Here's the drawing with two shaded views (mm, measured from the low corner). I have some questions. Give positions to 0.01 mm unless a question says otherwise; leave off trailing zeros. Write each loop counter-clockwise with the first axis right and the second up, starting at its lowest first coordinate (ties: lowest second). Pieces come first, ordered by that corner, then holes. Notation, with made-up numbers: M 72.25,22 L 102.25,22 A3 ccw 102.25,27 Z; hole C 76,88 d7. An arc over 180 degrees is marked long. Use one line per item in the form item = value.
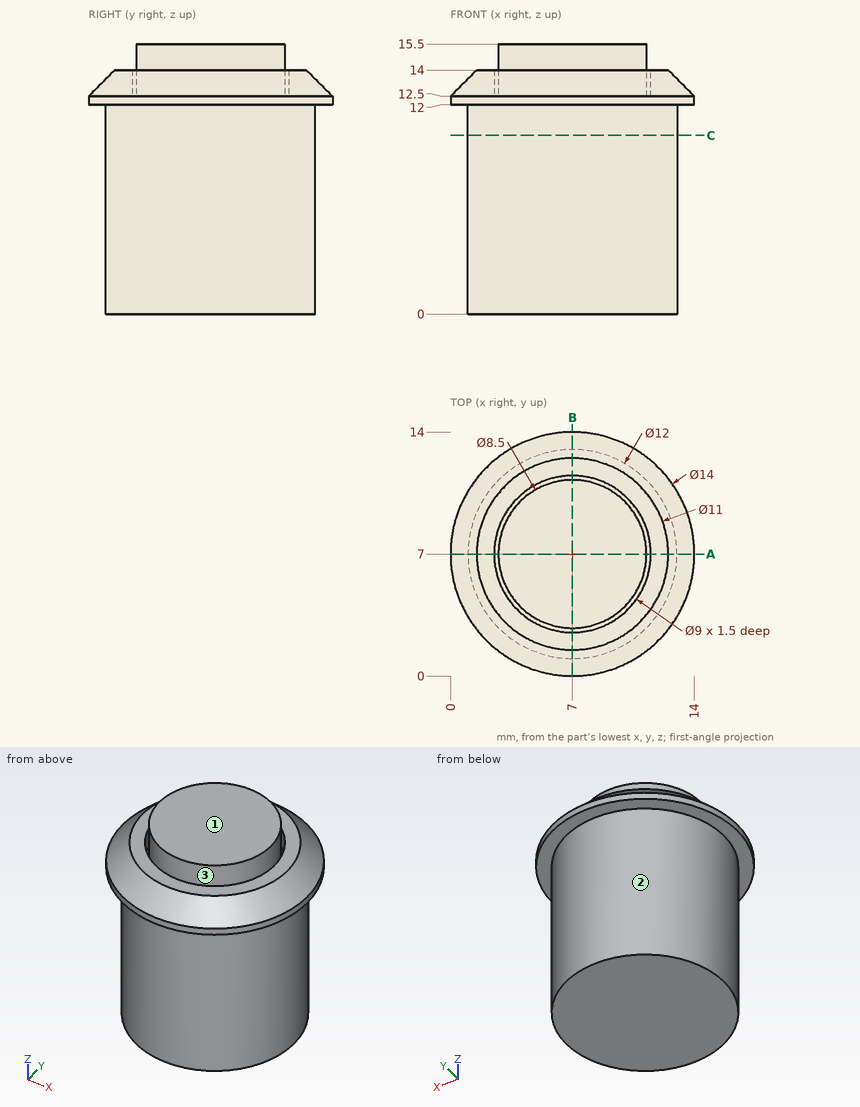
1) If I drill on L1, parallel to Y at x = 7, z = 13.15; L2, parallel to Y at x = 7, z = 12.95; L3, parallel to Z at x = 3, y = 4, over which ranges is the centre line in solid material (lowest first)?
Checked values:
L1 = 0.65 to 2.5, 2.75 to 11.25, 11.5 to 13.35
L2 = 0.45 to 2.5, 2.75 to 11.25, 11.5 to 13.55
L3 = 0 to 14
2) I want a section at A-A, the plane y = 7. Please give me the cut outline in (x, z).
Checked values:
outline = M 0,12 L 1,12 L 1,0 L 13,0 L 13,12 L 14,12 L 14,12.5 L 12.5,14 L 11.5,14 L 11.5,12.5 L 11.25,12.5 L 11.25,15.5 L 2.75,15.5 L 2.75,12.5 L 2.5,12.5 L 2.5,14 L 1.5,14 L 0,12.5 Z
3) I want a section at C-C, the plane z = 10.25. Please give me the cut outline in (x, y), plus the area to 3 significant figures.
Checked values:
outline = C 7,7 d12
area = 113 mm2
4) Thinking about a two-plate mould opening in X: for the marked faces 1, 2 and 3, which applies, released by +X, released by -X, zero draft, split by the parting line, or undercut?
Checked values:
face_1 = zero draft
face_2 = split by the parting line
face_3 = undercut
5) For pin 1 Ø1 at (y, z) = (2, 1.5) entering from +X; pin 2 Ø5 at (x, z) = (6.5, 7) entering from -Y; pin 3 Ø6 at (x, z) = (9.5, 4) entering from +Y, each with a flat end and sliding along its axis, tell me the tip position at first contact or that it passes through.
Checked values:
pin_1 = 10.97
pin_2 = 1
pin_3 = 13
